Check sheet for the modelled part. Datum: model origin and axes. Units: mm. Coordinates: 2 decimals unless noted, no trailing zeros. Write each loop counter-clockwise with the first axis right and the second up, starting at its lowest first coordinate (ties: lowest second). Pieces come first, ordered by that corner, then holes. Notation, with made-up numbers: M -20,43 L -13,43 A22 cw -13,67 Z; hole C 43,-18 d6. An arc over 180 degrees is marked long. Answer as CSV lines item,"result". Start each with the question number.
1) Material ranges on L1, parallel to Y at x = 0.25, z = 1.05; L2, parallel to Z at x = 2.75, y = -54; L3, parallel to Y at x = 3, z = 0.1, recorded low to high. Write a range as [from, to].
2) Section check B-B (y = -38). Record the cut outline in (x, z).
3) Go/stop test with flat-tipped pins: pin 1 Ø1 at (y, z) = (-63, 1) entering from +X; pin 2 Ø3 at (x, y) = (-2, -31.5) entering from +Z; pin 3 Ø1.5 at (x, z) = (2, 1) entering from -Y; pin 4 Ø0.8 at (y, z) = (2, -0.5) entering from +X. Record where each tip stops, or that it passes through.
from build123d import *

# Parameters (mm, degrees)
SKETCH1_W                = 4.5
SKETCH1_H                = 3.5
BOSS_EXTRUDE1_DEPTH      = 5
SKETCH2_W                = 3
SKETCH2_H                = 2
BOSS_EXTRUDE2_DEPTH      = 5.01
BOSS_EXTRUDE2_DEPTH_BACK = 0.01
FILLET2_R                = 0.5
SKETCH14_R               = 0.35


with BuildPart() as part:
    # Sketch1 → Boss-Extrude1 (new body)
    with BuildSketch(Plane(origin=(0, 0, 0), x_dir=(1, 0, 0), z_dir=(0, 1, 0))):
        Rectangle(SKETCH1_W, SKETCH1_H)
    extrude(amount=BOSS_EXTRUDE1_DEPTH)

    # Sketch2 → Boss-Extrude2 (add, two sides)
    with BuildSketch(Plane(origin=(0, 0, 0), x_dir=(1, 0, 0), z_dir=(0, 1, 0))) as boss_extrude2_sk:
        Rectangle(SKETCH2_W, SKETCH2_H)
    extrude(amount=BOSS_EXTRUDE2_DEPTH)
    extrude(boss_extrude2_sk.sketch, amount=-BOSS_EXTRUDE2_DEPTH_BACK)

    # Fillet2
    fillet2_edges = [part.edges().sort_by_distance(p)[0] for p in [
        (2.25, 2.5, 1.75),
        (-2.25, 2.5, 1.75),
        (-2.25, 2.5, -1.75),
        (2.25, 2.5, -1.75),
    ]]
    fillet(fillet2_edges, radius=FILLET2_R)

    # Sweep1: sweep along a path in Sketch15
    with BuildLine(Plane.XY) as sweep1_path:
        Line((2.25, 4.353782078), (2.3, 4.353782078))
        Line((2.3, 4.353782078), (2.525918375, 4.353782078))
        ThreePointArc((2.525918375, 4.353782078), (2.879471766, 4.207335469), (3.025918375, 3.853782078))
        Line((3.025918375, 3.853782078), (3.025918375, -71.146217922))
    # Sketch14 → Sweep1 (sweep)
    with BuildSketch(Plane(origin=(2.25, 0, 0), x_dir=(0, 0, -1), z_dir=(1, 0, 0))):
        with Locations((0, 4.353782078)):
            Circle(SKETCH14_R)
    sweep1 = sweep(path=sweep1_path.line)

    # Mirror1: Sweep1 across plane
    add(sweep1.mirror(Plane(origin=(0, 0, 0), x_dir=(0, 0, 1), z_dir=(1, 0, 0))))


solid = part.part
Results found:
1,L1,"y = [0, 5]"
1,L2,"z = [-0.22, 0.22]"
1,L3,"y = [-71.15, 4.54]"
2,outline,"C -3.03,0 d0.7; C 3.03,0 d0.7"
3,pin 1,"passes through"
3,pin 2,"stops at z = 0.35"
3,pin 3,"stops at y = -0.01"
3,pin 4,"stops at x = 3.36"
